```python
from build123d import *

# Parameters (mm, degrees)
F0_R     = 62.5
F0_R_2   = 17.25
F1_DEPTH = 14
F2_R     = 62.5
F2_R_2   = 33.5
F3_DEPTH = 1
F4_R     = 9.5
F5_DEPTH = 14.001


with BuildPart() as f1:
    # F0 (on Front) → F1 (new body)
    with BuildSketch(Plane.XZ):
        Circle(F0_R)
        Circle(F0_R_2, mode=Mode.SUBTRACT)
    extrude(amount=F1_DEPTH)

    # F2 (on face) → F3 (cut)
    with BuildSketch(Plane(origin=(0, 0, 0), x_dir=(-1, 0, 0), z_dir=(0, 1, 0))):
        Circle(F2_R)
        Circle(F2_R_2, mode=Mode.SUBTRACT)
    extrude(amount=-F3_DEPTH, mode=Mode.SUBTRACT)

    # F4 (on face) → F5 (cut, through all)
    with BuildSketch(Plane(origin=(0, 0, 0), x_dir=(-1, 0, 0), z_dir=(0, 1, 0))):
        with Locations((-31.819805, 31.819805)):
            Circle(F4_R)
        with Locations((-31.819805, -31.819805)):
            Circle(F4_R)
        with Locations((31.819805, -31.819805)):
            Circle(F4_R)
        with Locations((31.819805, 31.819805)):
            Circle(F4_R)
    extrude(amount=-F5_DEPTH, mode=Mode.SUBTRACT)


solid = f1.part
```
Geometry: final body of the model. Coordinates: model frame, mm. A direction names the side the tool comes from. Give positions to 0.01 mm unless a question says otherwise; leave off trailing zeros. Order: outer loops, then holes, each group sorted by start corner. A loop starts at its lowest first (then second) coordinate and runs counter-clockwise, first axis right, second up. Notation, with made-up numbers: (30, 72) -> (54, 72) arc R21 ccw to (54, 85) -> close; hole circle Ø10 at (48, 18.5). An arc over 180 degrees is marked (long way). Write each question's results on one line, items separated by ' | '. Start each with the question number.
1) Draft query along X for faces 3 (the cylindrical face through (-62.44, -7.41, 2.75)), 4 (the cylindrical face through (22.758, -7.409, 34.673)), 5 (the cylindrical face through (-24.28, -7.41, -37.6)), 6 (the flat face through (1, -1, -41)). Return one class per face: pulls with the +X half, pulls with the -X half, needs draft (parallel to the pull), parting line crosses it, or undercut.
2) First-contact query: pin 1 (2 mm diameter, centred on x = 44.5, y = -12, fed in from +Z); pin 2 (2 mm diameter, centred on x = 9.5, y = -12, fed in from +Z); pin 3 (1.5 mm diameter, centred on y = -7, z = -21, fed in from -X); pin 4 (15 mm diameter, centred on x = -31.82, z = -31.82, fed in from +Y). Flat tips, straight axial feed; report the tip coordinate or a pass-through.
3) Line query: line 1 (X direction, y = -6, z = 34.5); line 2 (X direction, y = -5.5, z = -30); line 3 (Z direction, x = 26, y = -10.5). Output: solid intervals per line, ascending. Write a range as from..to.
4) Section B-B (z = 0). Return loops of the section in (x, y), then the cut area to 3 significant figures.
5) Section C-C (z = -38.5). Return loops of the section in (x, y).
6) Section D-D (x = 25). Return loops of the section in (y, z), then the cut area to 3 significant figures.
7) Set-up query: faces 1 (the cylindrical face through (22.758, -7.409, -28.966)), 2 (the cylindrical face through (7.262, -0.493, -32.703)). Return all of +Z, -Z, +X, -X, +Y, -Y with unobstructed straight access to the full face (end or side cutting, diameter ignored); none if empty.
8) Section A-A (x = 0). Return loops of the section in (y, z).
Calculated:
1) face 3: parting line crosses it | face 4: undercut | face 5: undercut | face 6: needs draft
2) pin 1: z = 44.88 | pin 2: z = 61.92 | pin 3: x = -59.13 | pin 4: through
3) line 1: -52.12..-40.93, -22.71..22.71, 40.93..52.12 | line 2: -54.83..-41.14, -22.5..22.5, 41.14..54.83 | line 3: -56.84..-39.33, -24.31..24.31, 39.33..56.84
4) outline: (-62.5, -14) -> (-17.25, -14) -> (-17.25, 0) -> (-33.5, 0) -> (-33.5, -1) -> (-62.5, -1) -> close; (17.25, -14) -> (62.5, -14) -> (62.5, -1) -> (33.5, -1) -> (33.5, 0) -> (17.25, 0) -> close | area: 1,210 mm2
5) outline: (-49.23, -14) -> (-38.57, -14) -> (-38.57, -1) -> (-49.23, -1) -> close; (-25.07, -14) -> (25.07, -14) -> (25.07, -1) -> (-25.07, -1) -> close; (38.57, -14) -> (49.23, -14) -> (49.23, -1) -> (38.57, -1) -> close
6) outline: (-14, -57.28) -> (-1, -57.28) -> (-1, -38.43) -> (-14, -38.43) -> close; (-14, -25.21) -> (-1, -25.21) -> (-1, -22.3) -> (0, -22.3) -> (0, 22.3) -> (-1, 22.3) -> (-1, 25.21) -> (-14, 25.21) -> close; (-14, 38.43) -> (-1, 38.43) -> (-1, 57.28) -> (-14, 57.28) -> close | area: 1,190 mm2
7) face 1: +Y, -Y | face 2: +Y
8) outline: (-14, -62.5) -> (-1, -62.5) -> (-1, -33.5) -> (0, -33.5) -> (0, -17.25) -> (-14, -17.25) -> close; (-14, 17.25) -> (0, 17.25) -> (0, 33.5) -> (-1, 33.5) -> (-1, 62.5) -> (-14, 62.5) -> close
